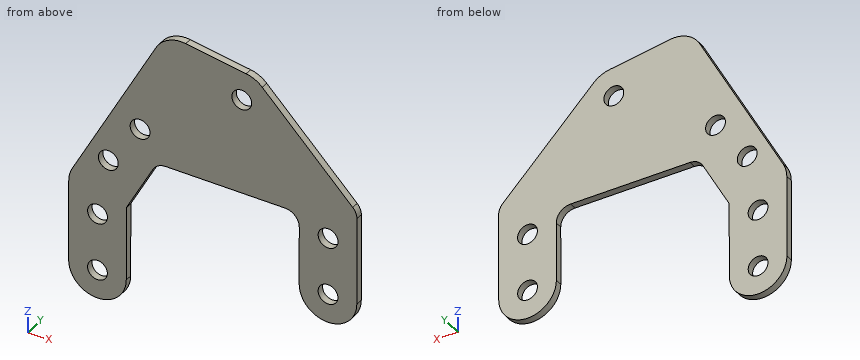
Autodesk Inventor part; units mm, degrees
ref_plane "YZ Plane" through (0, 0, 0) normal (1, 0, 0) x (0, 1, 0)
ref_plane "XZ Plane" through (0, 0, 0) normal (0, 1, 0) x (-1, 0, 0)
ref_plane "XY Plane" through (0, 0, 0) normal (0, 0, 1) x (1, 0, 0)
sketch "main" plane through (0, 0, 0) normal (0, 0, 1) x (1, 0, 0)
  circle A0 centre (12.325875, 33.112504) radius 2.1844
  line L0 (25.390984, 29.120631) -> (25.316771, 29.135118)
  line L1 (20.04973, 41.835118) -> (13.667964, 35.453352) construction
  arc A1 (20.04973, 41.835118) -> (17.011045, 41.065244) centre (20.04973, 35.453352) ccw
  circle A2 centre (25.38373, 35.485118) radius 2.1844
  line L2 (20.04973, 41.835118) -> (29.074911, 41.835118) construction
  arc A3 (25.38373, 41.835118) -> (25.38373, 41.835118) centre (25.38373, 35.485118) ccw
  circle A4 centre (12.68373, -15.314882) radius 2.1844
  circle A5 centre (-11.92252, 3.735118) radius 2.1844
  arc A6 (-18.198047, 2.765449) -> (-16.395825, -0.77177) centre (-11.92252, 3.735118) ccw
  line L3 (-20.257316, 16.092677) -> (-18.198047, 2.765449)
  line L4 (12.391865, -8.964882) -> (25.38373, -8.964882)
  circle A7 centre (25.38373, -15.314882) radius 2.1844
  arc A8 (25.38373, -21.664882) -> (25.38373, -8.964882) centre (25.38373, -15.314882) ccw
  line L5 (5.962319, -21.664882) -> (25.38373, -21.664882)
  line L6 (3.725666, -20.743326) -> (-16.395825, -0.77177)
  line L7 (21.760398, 29.194623) -> (10.880086, 23.303233)
  line L8 (-17.005348, 22.646303) -> (17.011045, 41.065244)
  circle A9 centre (2.776273, 26.136374) radius 2.1844
  arc A10 (-17.005348, 22.646303) -> (-20.257316, 16.092677) centre (-13.981788, 17.062345) ccw
  line L9 (9.216865, -5.789882) -> (9.216865, 20.511254)
  arc A11 (9.216865, -5.789882) -> (12.391865, -8.964882) centre (12.391865, -5.789882) ccw
  arc A12 (10.880086, 23.303233) -> (9.216865, 20.511254) centre (12.391865, 20.511254) ccw
  arc A13 (3.725666, -20.743326) -> (5.962319, -21.664882) centre (5.962319, -18.489882) ccw
  arc A14 (38.08373, 29.135118) -> (38.08373, 41.835118) centre (38.08373, 35.485118) ccw
  line L10 (20.04973, 41.835118) -> (38.08373, 41.835118)
  line L11 (21.650503, 29.135118) -> (38.08373, 29.135118)
  circle A15 centre (38.08373, 35.485118) radius 2.184401
  point P0 (7.427211, 10.378199)
  point P1 (19.03373, 40.819118)
  point P2 (-20.9407, 20.515419)
  point P3 (9.216865, -8.964882)
  point P4 (-30.17877, -11.346132)
  dimension "d0" = 4.3688
  dimension "d2" = 12.7
  dimension "d3" = 6.35
  dimension "d4" = 12.7
  dimension "d5" = 4.3688
  dimension "d6" = 4.3688
  dimension "d9" = 6.35
  dimension "d10" = 31.75
  dimension "d11" = 37.30625
  dimension "d16" = 6.35
  dimension "d18" = 3.175
  dimension "d21" = 4.7625
  dimension "d22" = 3.175
  dimension "d23" = 12.7
  dimension "d24" = 12.7
  dimension "d25" = 6.35
  dimension "d26" = 13.32723
sketch "Sketch1" plane through (0, 0, 0) normal (0, 1, 0) x (-1, 0, 0)
  circle A0 centre (-2.387595, 13.055125) radius 2.1844
  line L0 (-6.364475, -0.014556) -> (-6.350073, 0.059673)
  line L1 (6.343876, 5.341282) -> (-0.045209, 11.715722) construction
  arc A1 (6.343876, 5.341282) -> (5.570516, 8.379082) centre (-0.037886, 5.33396) ccw
  circle A2 centre (0, 0) radius 2.1844
  line L2 (6.343876, 5.341282) -> (6.354231, -3.683892) construction
  arc A3 (6.349996, 0.007286) -> (6.349996, 0.007286) centre (0, 0) ccw
  circle A4 centre (-50.814538, 12.641705) radius 2.1844
  circle A5 centre (-31.792784, 37.269796) radius 2.1844
  arc A6 (-32.769652, 43.544207) -> (-36.304801, 41.737927) centre (-31.792784, 37.269796) ccw
  line L3 (-19.444796, 45.618765) -> (-32.769652, 43.544207)
  line L4 (-44.464877, 12.940855) -> (-44.449971, -0.051001)
  circle A7 centre (-50.799967, -0.058287) radius 2.1844
  arc A8 (-57.149962, -0.065573) -> (-44.449971, -0.051001) centre (-50.799967, -0.058287) ccw
  line L5 (-57.172246, 19.355826) -> (-57.149962, -0.065573)
  line L6 (-56.253257, 21.593534) -> (-36.304801, 41.737927)
  line L7 (-6.294648, 3.616113) -> (-12.198518, 14.489658)
  line L8 (-12.887443, 42.374319) -> (5.570516, 8.379082)
  circle A9 centre (-9.374677, 22.596715) radius 2.1844
  arc A10 (-12.887443, 42.374319) -> (-19.444796, 45.618765) centre (-18.467928, 39.344355) ccw
  line L9 (-41.293522, 16.119496) -> (-14.992403, 16.149674)
  arc A11 (-41.293522, 16.119496) -> (-44.464877, 12.940855) centre (-41.289879, 12.944498) ccw
  arc A12 (-12.198518, 14.489658) -> (-14.992403, 16.149674) centre (-14.98876, 12.974676) ccw
  arc A13 (-56.253257, 21.593534) -> (-57.172246, 19.355826) centre (-53.997248, 19.359469) ccw
  arc A14 (-6.335424, -12.707278) -> (6.364568, -12.692706) centre (0.014572, -12.699992) ccw
  line L10 (6.343876, 5.341282) -> (6.364568, -12.692706)
  line L11 (-6.354279, 3.725939) -> (-6.335424, -12.707278)
  circle A15 centre (0.014572, -12.699992) radius 2.184401
  point P0 (0, 0)
extrude "Extrusion1" add sketch "Sketch1" along normal blind 1.5875
properties part number "Ring Funnel" material "Acetal Resin, White"
Can you work these out from the model? Positions are in its coordinate system, mm. Round coordinates to 2 decimals unless told otherwise and drop trailing zeros. Loops run counter-clockwise (first coordinate to the right, second up) from the corner with the lowest first, then second, coordinate; pieces in that order, holes last. Notation, with made-up numbers: (-17, 42) - (18, 42) arc R13 ccw to (18, 46) - close; hole circle Ø8 at (-0.75, 44.5). An arc over 180 degrees is marked (long way). Use CSV: the item, a comma, the result in double quotes. Start each with the question number.
1) Please list where these lines run through material, in increasing order: probe 1 along X at (y, z) = (1.3, 2.5); probe 2 along Z at (x, y) = (1, 0.9); probe 3 along Z at (x, y) = (-0.5, 0.25). Write a range as [from, to].
2) If we section it at C-C on z = 26: Write out the boundary of the cut face in (x, y).
3) If we section it at B-B on y = 0.95: Count the separate pieces of the cut face and the enclosed holes in it, plus the area to 3 significant figures.
4) If we section it at A-A on x = 10.5: Write out the boundary of the cut face in (y, z), plus the area to 3 significant figures.
5) If we section it at D-D on x = 40: Write out the boundary of the cut face in (y, z).
6) For pin 1 Ø5 at (x, z) = (0, 0) entering from +Y, with a flat end and sliding along its axis, tell me the tip position at first contact or that it passes through.
Geometry results:
1,probe 1,"x = [-6.35, 6.35], [44.45, 57.15]"
1,probe 2,"z = [-18.97, -14.63], [-10.77, -1.94], [1.94, 11.37], [14.74, 20.48]"
1,probe 3,"z = [-19.03, -14.83], [-10.57, -2.13], [2.13, 17.72]"
2,outline,"(4, 0) - (51.89, 0) - (51.89, 1.59) - (4, 1.59) - close"
3,separate pieces,"1"
3,enclosed holes,"7"
3,area,"1,780 mm2"
4,outline,"(0, 11.36) - (1.59, 11.36) - (1.59, 20.72) - (0, 20.72) - close; (0, 24.47) - (1.59, 24.47) - (1.59, 37.98) - (0, 37.98) - close"
4,area,"36.3 mm2"
5,outline,"(0, 16.12) - (1.59, 16.12) - (1.59, 38.01) - (0, 38.01) - close"
6,pin 1,"stops at y = 1.59"
